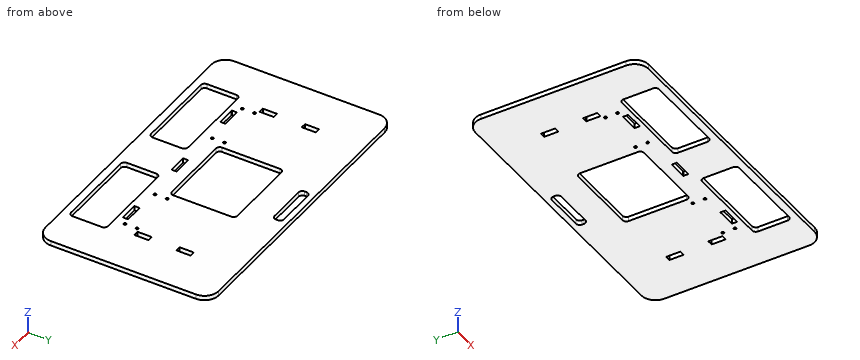
```python
from build123d import *

# Parameters (mm, degrees)
SKETCH_1_W                  = 640
SKETCH_1_H                  = 370
EXTRUDE_1618_DEPTH          = 5
SKETCH_2_W                  = 190
SKETCH_2_H                  = 79
CUT_EXTRUDE_1669_DEPTH      = 383.785840908
FILLET_R_R                  = 8
FILLET_R_OF_MIRROR_1948_R   = 8
CUT_EXTRUDE_1976_DEPTH      = 383.785840908
CUT_EXTRUDE_1976_DEPTH_BACK = 383.785840908
SKETCH_3_W                  = 170
SKETCH_3_H                  = 140
FILLET_R_2_R                = 8
SKETCH_4_W                  = 11.2
SKETCH_4_H                  = 30.4
CUT_EXTRUDE_2232_DEPTH      = 383.785840908
FILLET_R_3_R                = 0.5
FILLET_R_3_OF_MIRROR_2515_R = 0.5
MIRROR_START                = -5
MIRROR_2537_DEPTH           = 10
CUT_EXTRUDE_2565_DEPTH      = 383.785840908
CUT_EXTRUDE_2565_DEPTH_BACK = 383.785840908
SKETCH_5_W                  = 40.4
SKETCH_5_H                  = 11.2
FILLET_R_4_R                = 0.5
SKETCH_6_W                  = 40.4
SKETCH_6_H                  = 11.2
CUT_EXTRUDE_2821_DEPTH      = 383.785840908
FILLET_R_5_R                = 0.5
FILLET_R_5_OF_MIRROR_3088_R = 0.5
CUT_EXTRUDE_3116_DEPTH      = 383.785840908
CUT_EXTRUDE_3116_DEPTH_BACK = 383.785840908
SKETCH_7_W                  = 100
SKETCH_7_H                  = 20
FILLET_R_6_R                = 8
HOLE_WIZARD_3368_D          = 5.5
HOLE_WIZARD_3368_DEPTH      = 10
HOLE_WIZARD_3368_TIP        = 1.652366702
FILLET_R_7_R                = 30


# Read off the part's stored shape, not the designer's step: 角穴 筒受け・筒押え(後)
with BuildPart() as part:
    # ｽｹｯﾁ1 → Extrude 1618 (new, symmetric)
    with BuildSketch(Plane.XY):
        with Locations((0, -25)):
            Rectangle(SKETCH_1_W, SKETCH_1_H)
    extrude(amount=EXTRUDE_1618_DEPTH, both=True)

    # ｽｹｯﾁ2 → Cut-Extrude 1669 (cut, symmetric)
    with BuildSketch(Plane.XY):
        with Locations((140, -154.5)):
            Rectangle(SKETCH_2_W, SKETCH_2_H)
    cut_extrude_1669 = extrude(amount=CUT_EXTRUDE_1669_DEPTH, both=True, mode=Mode.SUBTRACT)

    # Fillet R
    fillet_r_edges = [part.edges().sort_by_distance(p)[0] for p in [
        (45, -194, 0),
        (45, -115, 0),
        (235, -115, 0),
        (235, -194, 0),
    ]]
    fillet(fillet_r_edges, radius=FILLET_R_R)

    # Mirror 1948: Cut-Extrude 1669 across plane
    add(cut_extrude_1669.mirror(Plane(origin=(0, 0, 0), x_dir=(0, 0, 1), z_dir=(1, 0, 0))), mode=Mode.SUBTRACT)

    # Fillet R of Mirror 1948
    fillet_r_of_mirror_1948_edges = [part.edges().sort_by_distance(p)[0] for p in [
        (-45, -194, 0),
        (-45, -115, 0),
        (-235, -115, 0),
        (-235, -194, 0),
    ]]
    fillet(fillet_r_of_mirror_1948_edges, radius=FILLET_R_OF_MIRROR_1948_R)

    # ｽｹｯﾁ3 → Cut-Extrude 1976 (cut, two sides: drawn at the far end of the back side and taken through both)
    with BuildSketch(Plane.XY.offset(-CUT_EXTRUDE_1976_DEPTH_BACK)):
        Rectangle(SKETCH_3_W, SKETCH_3_H)
    extrude(amount=CUT_EXTRUDE_1976_DEPTH + CUT_EXTRUDE_1976_DEPTH_BACK, mode=Mode.SUBTRACT)

    # Fillet R 2
    fillet_r_2_edges = [part.edges().sort_by_distance(p)[0] for p in [
        (-85, -70, 0),
        (-85, 70, 0),
        (85, 70, 0),
        (85, -70, 0),
    ]]
    fillet(fillet_r_2_edges, radius=FILLET_R_2_R)

    # ｽｹｯﾁ4 → Cut-Extrude 2232 (cut, symmetric)
    with BuildSketch(Plane.XY):
        with Locations((219, -45)):
            Rectangle(SKETCH_4_W, SKETCH_4_H)
    cut_extrude_2232 = extrude(amount=CUT_EXTRUDE_2232_DEPTH, both=True, mode=Mode.SUBTRACT)

    # Fillet R 3
    fillet_r_3_edges = [part.edges().sort_by_distance(p)[0] for p in [
        (213.4, -60.2, 0),
        (213.4, -29.8, 0),
        (224.6, -29.8, 0),
        (224.6, -60.2, 0),
    ]]
    fillet(fillet_r_3_edges, radius=FILLET_R_3_R)

    # Mirror 2515: Cut-Extrude 2232 across plane
    add(cut_extrude_2232.mirror(Plane.ZX), mode=Mode.SUBTRACT)

    # Fillet R 3 of Mirror 2515
    fillet_r_3_of_mirror_2515_edges = [part.edges().sort_by_distance(p)[0] for p in [
        (213.4, 60.2, 0),
        (213.4, 29.8, 0),
        (224.6, 29.8, 0),
        (224.6, 60.2, 0),
    ]]
    fillet(fillet_r_3_of_mirror_2515_edges, radius=FILLET_R_3_OF_MIRROR_2515_R)

    # Mirror 2537 outline → Mirror 2537 (cut)
    with BuildSketch(Plane.XY.offset(MIRROR_START)):
        with BuildLine():
            Line((-213.9, -29.8), (-224.1, -29.8))
            ThreePointArc((-224.1, -29.8), (-224.453553391, -29.946446609), (-224.6, -30.3))
            Line((-224.6, -30.3), (-224.6, -59.7))
            ThreePointArc((-224.6, -59.7), (-224.453553391, -60.053553391), (-224.1, -60.2))
            Line((-224.1, -60.2), (-213.9, -60.2))
            ThreePointArc((-213.9, -60.2), (-213.546446609, -60.053553391), (-213.4, -59.7))
            Line((-213.4, -59.7), (-213.4, -30.3))
            ThreePointArc((-213.4, -30.3), (-213.546446609, -29.946446609), (-213.9, -29.8))
        make_face()
        with BuildLine():
            ThreePointArc((-213.4, 59.7), (-213.546446609, 60.053553391), (-213.9, 60.2))
            Line((-213.9, 60.2), (-224.1, 60.2))
            ThreePointArc((-224.1, 60.2), (-224.453553391, 60.053553391), (-224.6, 59.7))
            Line((-224.6, 59.7), (-224.6, 30.3))
            ThreePointArc((-224.6, 30.3), (-224.453553391, 29.946446609), (-224.1, 29.8))
            Line((-224.1, 29.8), (-213.9, 29.8))
            ThreePointArc((-213.9, 29.8), (-213.546446609, 29.946446609), (-213.4, 30.3))
            Line((-213.4, 30.3), (-213.4, 59.7))
        make_face()
    extrude(amount=MIRROR_2537_DEPTH, mode=Mode.SUBTRACT)

    # ｽｹｯﾁ5 → Cut-Extrude 2565 (cut, two sides: drawn at the far end of the back side and taken through both)
    with BuildSketch(Plane.XY.offset(-CUT_EXTRUDE_2565_DEPTH_BACK)):
        with Locations((0, -100)):
            Rectangle(SKETCH_5_W, SKETCH_5_H)
    extrude(amount=CUT_EXTRUDE_2565_DEPTH + CUT_EXTRUDE_2565_DEPTH_BACK, mode=Mode.SUBTRACT)

    # Fillet R 4
    fillet_r_4_edges = [part.edges().sort_by_distance(p)[0] for p in [
        (-20.2, -105.6, 0),
        (-20.2, -94.4, 0),
        (20.2, -94.4, 0),
        (20.2, -105.6, 0),
    ]]
    fillet(fillet_r_4_edges, radius=FILLET_R_4_R)

    # ｽｹｯﾁ6 → Cut-Extrude 2821 (cut, symmetric)
    with BuildSketch(Plane.XY):
        with Locations((170, -100)):
            Rectangle(SKETCH_6_W, SKETCH_6_H)
    cut_extrude_2821 = extrude(amount=CUT_EXTRUDE_2821_DEPTH, both=True, mode=Mode.SUBTRACT)

    # Fillet R 5
    fillet_r_5_edges = [part.edges().sort_by_distance(p)[0] for p in [
        (149.8, -105.6, 0),
        (149.8, -94.4, 0),
        (190.2, -94.4, 0),
        (190.2, -105.6, 0),
    ]]
    fillet(fillet_r_5_edges, radius=FILLET_R_5_R)

    # Mirror 3088: Cut-Extrude 2821 across plane
    add(cut_extrude_2821.mirror(Plane(origin=(0, 0, 0), x_dir=(0, 0, 1), z_dir=(1, 0, 0))), mode=Mode.SUBTRACT)

    # Fillet R 5 of Mirror 3088
    fillet_r_5_of_mirror_3088_edges = [part.edges().sort_by_distance(p)[0] for p in [
        (-149.8, -105.6, 0),
        (-149.8, -94.4, 0),
        (-190.2, -94.4, 0),
        (-190.2, -105.6, 0),
    ]]
    fillet(fillet_r_5_of_mirror_3088_edges, radius=FILLET_R_5_OF_MIRROR_3088_R)

    # ｽｹｯﾁ7 → Cut-Extrude 3116 (cut, two sides: drawn at the far end of the back side and taken through both)
    with BuildSketch(Plane.XY.offset(-CUT_EXTRUDE_3116_DEPTH_BACK)):
        with Locations((0, 138)):
            Rectangle(SKETCH_7_W, SKETCH_7_H)
    extrude(amount=CUT_EXTRUDE_3116_DEPTH + CUT_EXTRUDE_3116_DEPTH_BACK, mode=Mode.SUBTRACT)

    # Fillet R 6
    fillet_r_6_edges = [part.edges().sort_by_distance(p)[0] for p in [
        (-50, 128, 0),
        (-50, 148, 0),
        (50, 148, 0),
        (50, 128, 0),
    ]]
    fillet(fillet_r_6_edges, radius=FILLET_R_6_R)

    # Hole Wizard 3368
    with Locations(Plane.XY.offset(5)):
        with Locations((100, -66), (100, -92), (-100, -66), (-100, -92), (205, -66), (205, -92), (-205, -66), (-205, -92)):
            Hole(HOLE_WIZARD_3368_D / 2, depth=HOLE_WIZARD_3368_DEPTH)
            with Locations((0, 0, -(HOLE_WIZARD_3368_DEPTH + HOLE_WIZARD_3368_TIP / 2))):  # 118° drill point
                Cone(0, HOLE_WIZARD_3368_D / 2, HOLE_WIZARD_3368_TIP, mode=Mode.SUBTRACT)

    # Fillet R 7
    fillet_r_7_edges = [part.edges().sort_by_distance(p)[0] for p in [
        (-320, 160, 0),
        (320, 160, 0),
        (320, -210, 0),
        (-320, -210, 0),
    ]]
    fillet(fillet_r_7_edges, radius=FILLET_R_7_R)


solid = part.part
```
Verification items for the finished model (mm, model axes). Coordinates: 2 decimals unless noted, no trailing zeros. Order: outer loops, then holes, each group sorted by start corner. A loop starts at its lowest first (then second) coordinate and runs counter-clockwise, first axis right, second up. Notation, with made-up numbers: (80.25, 33) -> (110.25, 33) arc R20 cw to (110.25, 58) -> close; hole circle Ø5 at (6, 0). An arc over 180 degrees is marked (long way). Answer as CSV lines item,"result". Start each with the question number.
1) Material ranges on L1, parallel to Y at x = 15, z = -0.75; L2, parallel to Y at x = 205, z = 1.25; L3, parallel to Y at x = 55.5, z = 2, recorded low to high. Write a range as [from, to].
2) Cross-section at A-A, the plane x = 177. Record the boundary of the cut face in (y, z).
3) Cross-section at B-B, the plane z = -0.5. Give the number of separate pieces and of enclosed holes in the cut face, then the cut area to 3 significant figures.
4) Gauge pin test, flat ends, axial feed: pin 1 Ø3.5 at (x, y) = (-205, -66) entering from -Z; pin 2 Ø2 at (y, z) = (139, -1.5) entering from -X. Record the tip position at first contact, or that the pin passes through.
Conclusion:
1,L1,"y = [-210, -105.6], [-94.4, -70], [70, 128], [148, 160]"
1,L2,"y = [-210, -194], [-115, -94.75], [-89.25, -68.75], [-63.25, 160]"
1,L3,"y = [-210, -194], [-115, -70], [70, 160]"
2,outline,"(-210, -5) -> (-194, -5) -> (-194, 5) -> (-210, 5) -> close; (-115, -5) -> (-105.6, -5) -> (-105.6, 5) -> (-115, 5) -> close; (-94.4, -5) -> (160, -5) -> (160, 5) -> (-94.4, 5) -> close"
3,separate pieces,"1"
3,enclosed holes,"19"
3,area,"178,000 mm²"
4,pin 1,"passes through"
4,pin 2,"stops at x = -318.91"
